from build123d import *

# Parameters (mm, degrees)
SKETCH_W      = 99.07
SKETCH_H      = 34.29
PAD_DEPTH     = 1.75
SKETCH001_R   = 1.365796
PAD001_DEPTH  = 2
SKETCH013_W   = 11.589402
SKETCH013_H   = 10.258059
SKETCH013_W_2 = 22.646941
SKETCH013_H_2 = 13.185007
PAD010_DEPTH  = 14
SKETCH016_W   = 9.758744
SKETCH016_H   = 10.16
PAD013_DEPTH  = 5.08
SKETCH017_W   = 10.16
SKETCH017_H   = 7.052728
PAD014_DEPTH  = 2.54


with BuildPart() as part:
    # Sketch → Pad (new body)
    with BuildSketch(Plane.XY):
        Rectangle(SKETCH_W, SKETCH_H)
    extrude(amount=PAD_DEPTH)

    # Sketch001 → Pad001 (join)
    with BuildSketch(Plane.XY):
        with Locations((-44.000565, 12.998089)):
            Circle(SKETCH001_R)
        with Locations((-22.000565, 12.999044)):
            Circle(SKETCH001_R)
        with Locations((-0.000565, 13)):
            Circle(SKETCH001_R)
        with Locations((21.999435, 13.000956)):
            Circle(SKETCH001_R)
        with Locations((43.999435, 13.001911)):
            Circle(SKETCH001_R)
        with Locations((-44, -0.001911)):
            Circle(SKETCH001_R)
        with Locations((-22, -0.000956)):
            Circle(SKETCH001_R)
        Circle(SKETCH001_R)
        with Locations((22, 0.000956)):
            Circle(SKETCH001_R)
        with Locations((44, 0.001911)):
            Circle(SKETCH001_R)
        with Locations((-43.999435, -13.001911)):
            Circle(SKETCH001_R)
        with Locations((-21.999435, -13.000956)):
            Circle(SKETCH001_R)
        with Locations((0.000565, -13)):
            Circle(SKETCH001_R)
        with Locations((22.000565, -12.999044)):
            Circle(SKETCH001_R)
        with Locations((44.000565, -12.998089)):
            Circle(SKETCH001_R)
    extrude(amount=-PAD001_DEPTH)

    # Sketch013 → Pad010 (join)
    with BuildSketch(Plane.XY.offset(1.75)):
        with Locations((-30.713279, 0.610479)):
            Rectangle(SKETCH013_W, SKETCH013_H)
        with Locations((19.642979, 1.424736)):
            Rectangle(SKETCH013_W_2, SKETCH013_H_2)
    extrude(amount=PAD010_DEPTH)

    # Sketch016 → Pad013 (join)
    with BuildSketch(Plane.XY.offset(1.75)):
        with Locations((48.238372, 7.62)):
            Rectangle(SKETCH016_W, SKETCH016_H)
        with Locations((48.238372, -7.62)):
            Rectangle(SKETCH016_W, SKETCH016_H)
    extrude(amount=PAD013_DEPTH)

    # Sketch017 → Pad014 (join)
    with BuildSketch(Plane.XY.offset(1.75)):
        with Locations((-39.372, 17.497364)):
            Rectangle(SKETCH017_W, SKETCH017_H)
        with Locations((-39.372, -17.497364)):
            Rectangle(SKETCH017_W, SKETCH017_H)
    extrude(amount=PAD014_DEPTH)


solid = part.part
Part model, mm, in its own coordinate system. A direction names the side the tool comes from. Coordinates: 2 decimals unless noted, no trailing zeros. Write each loop counter-clockwise with the first axis right and the second up, starting at its lowest first coordinate (ties: lowest second). Pieces come first, ordered by that corner, then holes. Notation, with made-up numbers: M -21,44 L 7,44 A17 ccw 7,73 Z; hole C -3,28 d9. An arc over 180 degrees is marked long. Return JSON: item names as keys, results as strings.
1. Pull direction X, two halves, no side cores. Call faces 5 (the face through (20.99, -12.08, -0.99)), 6 (the face through (22, 0, -2)): pulls with the +X half, pulls with the -X half, needs draft (parallel to the pull), parting line crosses it, or undercut.
Determined:
{"face 5": "undercut", "face 6": "needs draft"}
2. Saw through at A-A, the plane x = 17. Write the cut outline in (y, z) (3 decimals).
Determined:
{"outline": "M -17.145,0 L 17.145,0 L 17.145,1.75 L 8.017,1.75 L 8.017,15.75 L -5.168,15.75 L -5.168,1.75 L -17.145,1.75 Z"}
3. Saw through at B-B, the plane z = 14.25. Write the cut outline in (x, y), then the cut area to 3 significant figures.
Determined:
{"outline": "M -36.51,-4.52 L -24.92,-4.52 L -24.92,5.74 L -36.51,5.74 Z; M 8.32,-5.17 L 30.97,-5.17 L 30.97,8.02 L 8.32,8.02 Z", "area": "417 mm²"}
4. 3-axis set-ups, long thin cutter, end or side, ignore diameter. For faces 1 (the face through (19, 8.017, 9)), 2 (the face through (-39, -17, 4.29)), 3 (the face through (-39, 19, 1.75)), 4 (the face through (-23.364, 0.059, -0.986)): which of +Z, -Z, +X, -X, +Y, -Y reach the whole face in a straight line?
Determined:
{"face 1": "+Z, -X, +Y", "face 2": "+Z, +X, -X, -Y", "face 3": "-Z, +X, -X, +Y", "face 4": "-Z"}
5. Saw through at C-C, the plane y = -16. Write the cut outline in (x, z) (3 decimals), then the cut area to 3 significant figures.
Determined:
{"outline": "M -49.535,0 L 49.535,0 L 49.535,1.75 L -34.292,1.75 L -34.292,4.29 L -44.452,4.29 L -44.452,1.75 L -49.535,1.75 Z", "area": "199 mm²"}
6. Flat gauge pins, fed straight in: pin 1 Ø8 at (x, y) = (-41, -17.5) entering from +Z; pin 2 Ø2.5 at (x, z) = (46, 5) entering from +Y; pin 3 Ø6 at (x, y) = (-28.5, -4) entering from -Z. Where does each tip first touch, or does it go through?
Determined:
{"pin 1": "z = 4.29", "pin 2": "y = 12.7", "pin 3": "z = 0"}
7. Probe L1, parallel to X at y = 4, z = 3.5; L2, parallel to Y at x = 44.5, z = -1; L3, parallel to Y at x = -39, z = 2.75. List the from-to ranges inside material, lowest first.
Determined:
{"L1": "-36.51 to -24.92, 8.32 to 30.97, 43.36 to 53.12", "L2": "-14.27 to -11.73, -1.27 to 1.27, 11.73 to 14.27", "L3": "-21.02 to -13.97, 13.97 to 21.02"}
8. Saw through at D-D, the plane x = -22. Write the cut outline in (y, z) (3 decimals).
Determined:
{"outline": "M -17.145,0 L -14.367,0 L -14.367,-2 L -11.635,-2 L -11.635,0 L -1.367,0 L -1.367,-2 L 1.365,-2 L 1.365,0 L 11.633,0 L 11.633,-2 L 14.365,-2 L 14.365,0 L 17.145,0 L 17.145,1.75 L -17.145,1.75 Z"}
